from build123d import *

# Parameters (mm, degrees)
F0_W     = 215.9
F0_H     = 206.375
F1_DEPTH = 57.15
F2_T     = -3.175
F3_W     = 203.2
F3_H     = 3.175
F4_DEPTH = 3.175
F5_W     = 203.2
F5_H     = 3.175
F6_DEPTH = 3.175


with BuildPart() as f1:
    # F0 (on Top) → F1 (new body)
    with BuildSketch(Plane.XY):
        Rectangle(F0_W, F0_H)
    extrude(amount=F1_DEPTH)

    # F2
    f2_openings = [f1.faces().sort_by_distance(p)[0] for p in [
        (0, -103.1875, 28.575),
    ]]
    offset(amount=F2_T, openings=f2_openings)

    # F3 (on face) → F4 (join)
    with BuildSketch(Plane.YZ.offset(-104.775)):
        with Locations((-1.5875, 40.2166666663)):
            Rectangle(F3_W, F3_H)
        with Locations((-1.5875, 33.8666666663)):
            Rectangle(F3_W, F3_H)
        with Locations((-1.5875, 23.2833333337)):
            Rectangle(F3_W, F3_H)
        with Locations((-1.5875, 16.9333333337)):
            Rectangle(F3_W, F3_H)
    extrude(amount=F4_DEPTH)

    # F5 (on face) → F6 (join)
    with BuildSketch(Plane(origin=(104.775, 0, 0), x_dir=(0, -1, 0), z_dir=(-1, 0, 0))):
        with Locations((1.5875, 40.2166666663)):
            Rectangle(F5_W, F5_H)
        with Locations((1.5875, 33.8666666663)):
            Rectangle(F5_W, F5_H)
        with Locations((1.5875, 23.2833333337)):
            Rectangle(F5_W, F5_H)
        with Locations((1.5875, 16.9333333337)):
            Rectangle(F5_W, F5_H)
    extrude(amount=F6_DEPTH)


solid = f1.part
CAD build for the part. Positions are in the model's coordinates, mm. A direction names the side the tool comes from. Give positions to 0.01 mm unless a question says otherwise; leave off trailing zeros. Return JSON: item names as keys, results as strings.
Item 1: Drop flat-ended pins along their axis: pin 1 (6 mm diameter, centred on x = -22, z = 36, fed in from -Y); pin 2 (2.5 mm diameter, centred on x = 103.5, y = 42, fed in from -Z). Give the stop position or say it passes through.
Answer below:
{"pin 1": "stops at y = 100.01", "pin 2": "stops at z = 0"}
Item 2: Drill centre lines: probe 1 along X at (y, z) = (10, 52) (3 decimals); probe 2 along Z at (x, y) = (39.5, 1) (3 decimals); probe 3 along X at (y, z) = (6.5, 16). Where is each one in solid material? Low to high.
Answer below:
{"probe 1": "x = -107.95 to -104.775, 104.775 to 107.95", "probe 2": "z = 0 to 3.175, 53.975 to 57.15", "probe 3": "x = -107.95 to -101.6, 101.6 to 107.95"}
Item 3: Tool access for faces 1 (the flat face through (104.775, -3, 9)), 2 (the flat face through (-2, 1, 57.15)): list every direction of +Z, -Z, +X, -X, +Y, -Y with a clear straight run to the whole face (end or side of a thin tool).
Answer below:
{"face 1": "-Y", "face 2": "+Z, +X, -X, +Y, -Y"}
